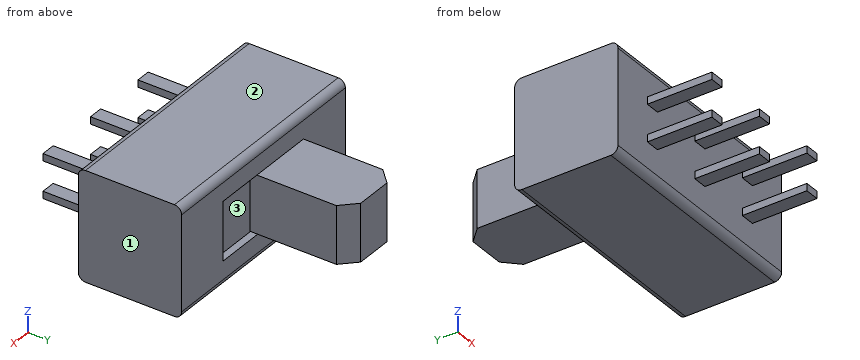
Autodesk Inventor part; units mm, degrees
ref_plane "YZ Plane" through (0, 0, 0) normal (1, 0, 0) x (0, 1, 0)
ref_plane "XZ Plane" through (0, 0, 0) normal (0, 1, 0) x (-1, 0, 0)
ref_plane "XY Plane" through (0, 0, 0) normal (0, 0, 1) x (1, 0, 0)
sketch "Sketch1" plane through (0, 0, 0) normal (0, 1, 0) x (-1, 0, 0)
  line L0 (17.8833, -8.321) -> (1.6833, -8.321)
  line L1 (1.6833, -8.321) -> (1.6833, -0.721)
  line L2 (1.6833, -0.721) -> (17.8833, -0.721)
  line L3 (17.8833, -0.721) -> (17.8833, -8.321)
  dimension "d23" = 16.2
extrude "Extrusion5" add sketch "Sketch1" along normal blind 7.2
fillet "Fillet2" radius 0.5 4 edges at (-9.7833, 7.2, -0.721) (-9.7833, 7.2, -8.321) (-9.7833, 0, -0.721) (-9.7833, 0, -8.321)
sketch "Sketch7" plane through (0, 7.2, 0) normal (0, 1, 0) x (1, 0, 0)
  line L0 (-17.8833, 7.821) -> (-1.6833, 7.821)
  line L1 (-17.8833, 7.821) -> (-17.8833, 1.221)
  line L2 (-1.6833, 1.221) -> (-17.8833, 1.221)
  line L3 (-1.6833, 1.221) -> (-1.6833, 7.821)
  line L4 (-13.8133, 2.491) -> (-5.7533, 2.491)
  line L5 (-5.7533, 2.491) -> (-5.7533, 6.551)
  line L6 (-5.7533, 6.551) -> (-13.8133, 6.551)
  line L7 (-13.8133, 6.551) -> (-13.8133, 2.491)
  line L8 (-13.8133, 2.491) -> (-5.7533, 6.551) construction
  line L9 (-5.7533, 2.491) -> (-13.8133, 6.551) construction
  point P0 (0, 0)
  point P1 (-9.7833, 4.521)
  dimension "d28" = 8.06
  dimension "d29" = 4.06
extrude "Extrusion6" cut sketch "Sketch7" against normal blind 0.5 contours L7 L6 L5 L4
sketch "Sketch8" plane through (0, 6.7, 0) normal (0, 1, 0) x (1, 0, 0)
  line L0 (-13.7727, 6.521) -> (-9.1727, 6.521)
  line L1 (-9.1727, 6.521) -> (-9.1727, 2.521)
  line L2 (-9.1727, 2.521) -> (-13.7727, 2.521)
  line L3 (-13.7727, 2.521) -> (-13.7727, 6.521)
  line L4 (-13.7727, 6.521) -> (-9.1727, 2.521) construction
  line L5 (-9.1727, 6.521) -> (-13.7727, 2.521) construction
  line L6 (-13.8133, 6.551) -> (-5.7533, 6.551)
  line L7 (-13.8133, 2.491) -> (-13.8133, 6.551)
  line L8 (-5.7533, 2.491) -> (-13.8133, 2.491)
  line L9 (-5.7533, 6.551) -> (-5.7533, 2.491)
  point P0 (0, 0)
  point P1 (-11.4727, 4.521)
  dimension "d32" = 4.6
  dimension "d33" = 4
  dimension "d34" = 2.03
extrude "Extrusion7" add sketch "Sketch8" along normal blind 7 contours L0 L1 L2 L3
chamfer "Chamfer1" distance 1 angle 45 2 edges at (-9.1727, 13.7, -4.521) (-13.7727, 13.7, -4.521)
sketch "Sketch9" plane through (0, 0, 0) normal (0, -1, 0) x (1, 0, 0)
  line L0 (-1.6833, -7.821) -> (-17.8833, -7.821)
  line L1 (-1.6833, -1.221) -> (-1.6833, -7.821)
  line L2 (-17.8833, -1.221) -> (-1.6833, -1.221)
  line L3 (-17.8833, -7.821) -> (-17.8833, -1.221)
  line L4 (-5.5833, -2.991) -> (-4.5833, -2.991)
  line L5 (-4.5833, -2.991) -> (-4.5833, -3.491)
  line L6 (-4.5833, -3.491) -> (-5.5833, -3.491)
  line L7 (-5.5833, -3.491) -> (-5.5833, -2.991)
  line L8 (-5.5833, -2.991) -> (-4.5833, -3.491) construction
  line L9 (-4.5833, -2.991) -> (-5.5833, -3.491) construction
  line L10 (-10.2833, -2.991) -> (-9.2833, -2.991)
  line L11 (-9.2833, -2.991) -> (-9.2833, -3.491)
  line L12 (-9.2833, -3.491) -> (-10.2833, -3.491)
  line L13 (-10.2833, -3.491) -> (-10.2833, -2.991)
  line L14 (-10.2833, -2.991) -> (-9.2833, -3.491) construction
  line L15 (-9.2833, -2.991) -> (-10.2833, -3.491) construction
  line L16 (-14.9833, -2.991) -> (-13.9833, -2.991)
  line L17 (-13.9833, -2.991) -> (-13.9833, -3.491)
  line L18 (-13.9833, -3.491) -> (-14.9833, -3.491)
  line L19 (-14.9833, -3.491) -> (-14.9833, -2.991)
  line L20 (-14.9833, -2.991) -> (-13.9833, -3.491) construction
  line L21 (-13.9833, -2.991) -> (-14.9833, -3.491) construction
  line L22 (-5.5833, -5.551) -> (-4.5833, -5.551)
  line L23 (-4.5833, -5.551) -> (-4.5833, -6.051)
  line L24 (-4.5833, -6.051) -> (-5.5833, -6.051)
  line L25 (-5.5833, -6.051) -> (-5.5833, -5.551)
  line L26 (-5.5833, -5.551) -> (-4.5833, -6.051) construction
  line L27 (-4.5833, -5.551) -> (-5.5833, -6.051) construction
  line L28 (-10.2833, -5.551) -> (-9.2833, -5.551)
  line L29 (-9.2833, -5.551) -> (-9.2833, -6.051)
  line L30 (-9.2833, -6.051) -> (-10.2833, -6.051)
  line L31 (-10.2833, -6.051) -> (-10.2833, -5.551)
  line L32 (-10.2833, -5.551) -> (-9.2833, -6.051) construction
  line L33 (-9.2833, -5.551) -> (-10.2833, -6.051) construction
  line L34 (-14.9833, -5.551) -> (-13.9833, -5.551)
  line L35 (-13.9833, -5.551) -> (-13.9833, -6.051)
  line L36 (-13.9833, -6.051) -> (-14.9833, -6.051)
  line L37 (-14.9833, -6.051) -> (-14.9833, -5.551)
  line L38 (-14.9833, -5.551) -> (-13.9833, -6.051) construction
  line L39 (-13.9833, -5.551) -> (-14.9833, -6.051) construction
  line L40 (-1.6833, -1.221) -> (-17.8833, -1.221)
  line L41 (-9.7833, -1.221) -> (-9.7833, -7.821) construction
  line L42 (-17.8833, -7.821) -> (-1.6833, -7.821)
  line L43 (-1.6833, -1.221) -> (-1.6833, -7.821)
  line L44 (-1.6833, -4.521) -> (-17.8833, -4.521) construction
  line L45 (-17.8833, -7.821) -> (-17.8833, -1.221)
  point P0 (0, 0)
  point P1 (-5.0833, -3.241)
  point P2 (-9.7833, -3.241)
  point P3 (-14.4833, -3.241)
  point P4 (-5.0833, -5.801)
  point P5 (-9.7833, -5.801)
  point P6 (-14.4833, -5.801)
  point P7 (-9.7833, -3.241)
  dimension "d40" = 1
  dimension "d41" = 0.5
  dimension "d44" = 4.7
  dimension "d47" = 2.56
  dimension "d50" = 1.28
extrude "Extrusion8" add sketch "Sketch9" along normal blind 4.5 contours L4 L5 L6 L7 | L10 L11 L12 L13 | L16 L17 L18 L19 | L22 L23 L24 L25 | L28 L29 L30 L31 | L34 L35 L36 L37
properties part number "switch" material "PAEK Plastic"
Model file for the job. Use its own axes, mm. Face numbers are marked on the shaded views. Give positions to 0.01 mm unless a question says otherwise; leave off trailing zeros. Order: outer loops, then holes, each group sorted by start corner. A loop starts at its lowest first (then second) coordinate and runs counter-clockwise, first axis right, second up. Notation, with made-up numbers: (54.5, 64) -> (61.5, 64) arc R31 cw to (61.5, 102) -> close; hole circle Ø10 at (0.5, 28). An arc over 180 degrees is marked (long way). Use CSV: the item, a comma, the result in double quotes.
1. Band-saw the part on C-C, the plane z = -4.75. Give the cut face in (x, y).
Outcome:
outline,"(-17.88, 0) -> (-1.68, 0) -> (-1.68, 7.2) -> (-5.75, 7.2) -> (-5.75, 6.7) -> (-9.17, 6.7) -> (-9.17, 12.7) -> (-10.17, 13.7) -> (-12.77, 13.7) -> (-13.77, 12.7) -> (-13.77, 6.7) -> (-13.81, 6.7) -> (-13.81, 7.2) -> (-17.88, 7.2) -> close"
2. Band-saw the part on A-A, the plane y = -2. Give the cut face in (x, z), then the cut area to 3 significant figures.
Outcome:
outline,"(-14.98, -6.05) -> (-13.98, -6.05) -> (-13.98, -5.55) -> (-14.98, -5.55) -> close; (-14.98, -3.49) -> (-13.98, -3.49) -> (-13.98, -2.99) -> (-14.98, -2.99) -> close; (-10.28, -6.05) -> (-9.28, -6.05) -> (-9.28, -5.55) -> (-10.28, -5.55) -> close; (-10.28, -3.49) -> (-9.28, -3.49) -> (-9.28, -2.99) -> (-10.28, -2.99) -> close; (-5.58, -6.05) -> (-4.58, -6.05) -> (-4.58, -5.55) -> (-5.58, -5.55) -> close; (-5.58, -3.49) -> (-4.58, -3.49) -> (-4.58, -2.99) -> (-5.58, -2.99) -> close"
area,"3.00 mm²"
3. Drop flat-ended pins along their axis: pin 1 (1.2 mm diameter, centred on y = 10.5, z = -5, fed in from -X); pin 2 (0.8 mm diameter, centred on x = -10, y = -3, fed in from -Z); pin 3 (1.4 mm diameter, centred on x = -12, y = 10.5, fed in from +Z). Give the stop position or say it passes through.
Outcome:
pin 1,"x = -13.77"
pin 2,"z = -6.05"
pin 3,"z = -2.52"
4. Mould opens along Z. For the marked faces 1, 2 and 3 say: +Z half, -Z half, draft (parallel to the pull), parting line (faces both ways), or undercut.
Outcome:
face 1,"draft"
face 2,"+Z half"
face 3,"undercut"
5. Drill centre lines: line 1 along X through (y, z) = (-2.25, -5.75); line 2 along X through (y, z) = (9.75, -5.25); line 3 along Y through (x, z) = (-11.75, -5). Where is each one in solid material? Low to high. Write a range as from..to.
Outcome:
line 1,"-14.98..-13.98, -10.28..-9.28, -5.58..-4.58"
line 2,"-13.77..-9.17"
line 3,"0..13.7"
6. Band-saw the part on B-B, the plane x = -6.75. Give the cut face in (y, z).
Outcome:
outline,"(0, -7.82) arc R0.5 ccw to (0.5, -8.32) -> (6.7, -8.32) arc R0.5 ccw to (7.2, -7.82) -> (7.2, -6.55) -> (6.7, -6.55) -> (6.7, -2.49) -> (7.2, -2.49) -> (7.2, -1.22) arc R0.5 ccw to (6.7, -0.72) -> (0.5, -0.72) arc R0.5 ccw to (0, -1.22) -> close"
